from build123d import *

# Parameters (mm, degrees)
SKETCH1_W           = 14
SKETCH1_H           = 26
SKETCH1_R           = 0.5
SKETCH1_R_2         = 0.4
SKETCH1_R_3         = 1.55
BOSS_EXTRUDE1_DEPTH = 1.6
CHAMFER1_SIZE       = 1


with BuildPart() as part:
    # Sketch1 → Boss-Extrude1 (new body)
    with BuildSketch(Plane.XY):
        with Locations((0, 13)):
            Rectangle(SKETCH1_W, SKETCH1_H)
        with Locations((-0.04, 23.5)):
            Circle(SKETCH1_R, mode=Mode.SUBTRACT)
        with Locations((2.5, 23.5)):
            Circle(SKETCH1_R, mode=Mode.SUBTRACT)
        with Locations((5.04, 23.5)):
            Circle(SKETCH1_R, mode=Mode.SUBTRACT)
        with Locations((-5.04, 2.05)):
            Circle(SKETCH1_R_2, mode=Mode.SUBTRACT)
        with Locations((-3.77, 2.05)):
            Circle(SKETCH1_R_2, mode=Mode.SUBTRACT)
        with Locations((-1.23, 2.05)):
            Circle(SKETCH1_R_2, mode=Mode.SUBTRACT)
        with Locations((0.04, 2.05)):
            Circle(SKETCH1_R_2, mode=Mode.SUBTRACT)
        with Locations((3.7, 7)):
            Circle(SKETCH1_R_3, mode=Mode.SUBTRACT)
        with Locations((3.7, 17)):
            Circle(SKETCH1_R_3, mode=Mode.SUBTRACT)
    extrude(amount=BOSS_EXTRUDE1_DEPTH)

    # Chamfer1
    chamfer1_edges = [part.edges().sort_by_distance(p)[0] for p in [
        (-7, 26, 0.8),
    ]]
    chamfer(chamfer1_edges, length=CHAMFER1_SIZE)


solid = part.part
Geometry: final body of the model. Coordinates: model frame, mm. Round coordinates to 2 decimals unless told otherwise and drop trailing zeros. Order: outer loops, then holes, each group sorted by start corner. A loop starts at its lowest first (then second) coordinate and runs counter-clockwise, first axis right, second up. Notation, with made-up numbers: (-11, 65.25) -> (44, 65.25) arc R13 ccw to (44, 78.25) -> close; hole circle Ø10 at (22, 0.5). An arc over 180 degrees is marked (long way). Put each result on its own line as item: value. Start each with the question number.
Q1. Pull-direction query (Y, two-part tool) for faces 1 (the flat face through (0, 13, 1.6)), 2 (the flat face through (-6.5, 25.5, 0.8)), 3 (the cylindrical face through (0, 24, 1)); classes: +Y half, -Y half, draft (parallel to the pull), parting line (faces both ways), or undercut.
Q2. Section A-A on x = -0.04. Return the cut outline in (y, z).
Q3. First-contact query: pin 1 (2.5 mm diameter, centred on x = 3.7, y = 7, fed in from +Z). Flat tip, straight axial feed; report the tip coordinate or a pass-through.
Q4. Section D-D on x = -3.77. Return the cut outline in (y, z), and give its area (3 significant figures).
Q5. Section C-C on z = 0.5. Give the number of separate pieces and of enclosed holes in the cut face, and give its area (3 significant figures).
Q6. Line query: probe 1 along Y at (x, z) = (3.75, 0.7); probe 2 along Y at (x, z) = (-5.04, 0.5); probe 3 along Y at (x, z) = (4.5, 0.5). Output: solid intervals per line, ascending.
Q7. Section B-B on y = 7. Return the cut outline in (x, z).
Ans:
1. face 1: draft
1. face 2: +Y half
1. face 3: undercut
2. outline: (0, 0) -> (1.66, 0) -> (1.66, 1.6) -> (0, 1.6) -> close; (2.44, 0) -> (23, 0) -> (23, 1.6) -> (2.44, 1.6) -> close; (24, 0) -> (26, 0) -> (26, 1.6) -> (24, 1.6) -> close
3. pin 1: passes through
4. outline: (0, 0) -> (1.65, 0) -> (1.65, 1.6) -> (0, 1.6) -> close; (2.45, 0) -> (26, 0) -> (26, 1.6) -> (2.45, 1.6) -> close
4. area: 40.3 mm2
5. separate pieces: 1
5. enclosed holes: 9
5. area: 344 mm2
6. probe 1: y = 0 to 5.45, 8.55 to 15.45, 18.55 to 26
6. probe 2: y = 0 to 1.65, 2.45 to 26
6. probe 3: y = 0 to 5.67, 8.33 to 15.67, 18.33 to 26
7. outline: (-7, 0) -> (2.15, 0) -> (2.15, 1.6) -> (-7, 1.6) -> close; (5.25, 0) -> (7, 0) -> (7, 1.6) -> (5.25, 1.6) -> close
